Geometry check sheet. Reference: drawing and pictorial views, mm from the part's lowest x, y, z. Coordinates: 2 decimals unless noted, no trailing zeros. Loops run counter-clockwise (first coordinate to the right, second up) from the corner with the lowest first, then second, coordinate; pieces in that order, holes last. Notation, with made-up numbers: (76.25, -1.75) -> (123.25, -1.75) arc R15 ccw to (123.25, 9.25) -> close; hole circle Ø5 at (88, -30). An arc over 180 degrees is marked (long way). Use one line per item in the form item = value.
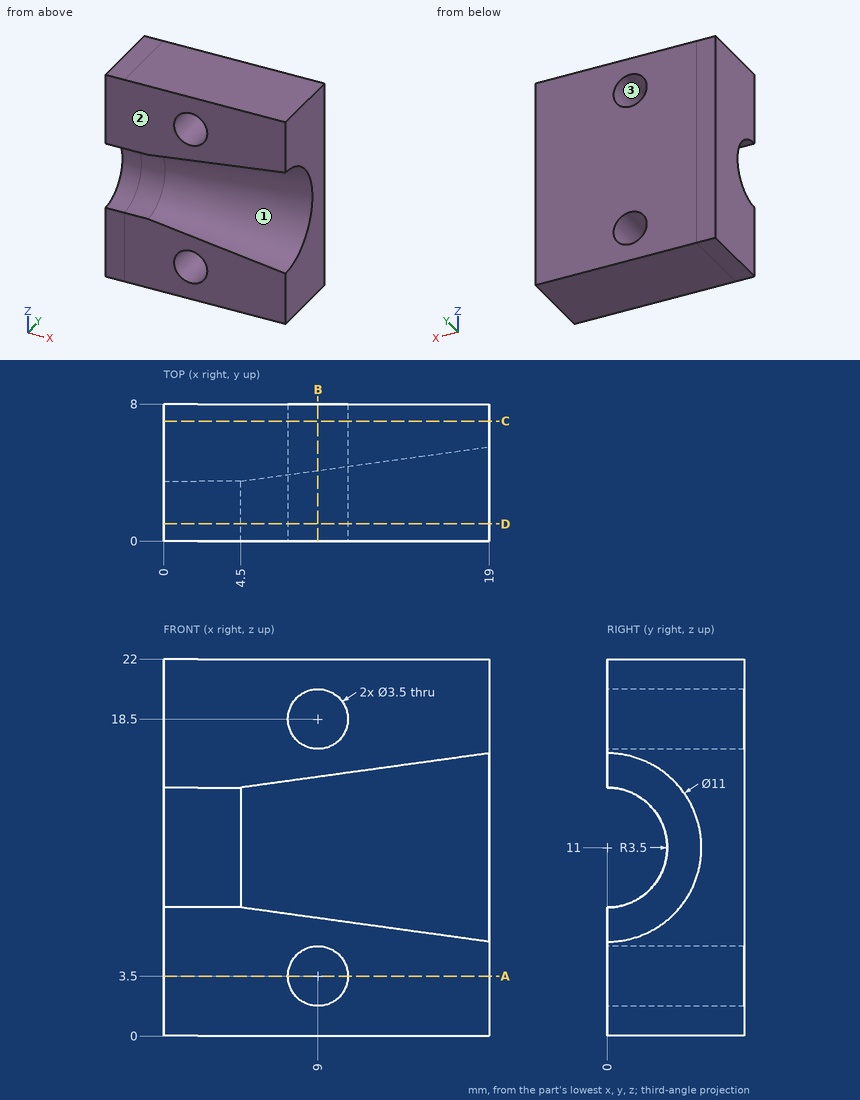
(1) Scan lines: line 1 along Z through (x, y) = (9, 5.75); line 2 along Z through (x, y) = (9.5, 2.5); line 3 along Z through (x, y) = (9, 3). Record each from-to range of solid material in increasing order.
Established:
line_1 = 0 to 1.75, 5.25 to 16.75, 20.25 to 22
line_2 = 0 to 1.82, 5.18 to 7.64, 14.36 to 16.82, 20.18 to 22
line_3 = 0 to 1.75, 5.25 to 8.18, 13.82 to 16.75, 20.25 to 22
(2) Section check D-D, the plane y = 1. Give the number of separate pieces and of enclosed holes in the cut face, plus the area to 3 significant figures.
Established:
separate_pieces = 2
enclosed_holes = 2
area = 241 mm²
(3) Mould release check, pull along X, two halves, no side actions. Record for the marked faces 1, 2 and 3: +X half, -X half, draft (parallel to the pull), parting line (faces both ways), or undercut.
Established:
face_1 = +X half
face_2 = draft
face_3 = undercut
(4) Section check A-A, the plane z = 3.5. Record the boundary of the cut face in (x, y).
Established:
outline = (0, 0) -> (7.25, 0) -> (7.25, 8) -> (0, 8) -> close; (10.75, 0) -> (19, 0) -> (19, 8) -> (10.75, 8) -> close
(5) Go/stop test with flat-tipped pins: P1, Ø4, axis at x = 2.5, z = 10.5, coming from the -Y side; P2, Ø3, axis at x = 9, z = 18.5, coming from the -Y side. Record where each tip stops, or that it passes through.
Established:
P1 = 2.45
P2 = through
(6) Section check C-C, the plane y = 7. Record the boundary of the cut face in (x, z), plus the area to 3 significant figures.
Established:
outline = (0, 0) -> (19, 0) -> (19, 22) -> (0, 22) -> close; hole circle Ø3.5 at (9, 3.5); hole circle Ø3.5 at (9, 18.5)
area = 399 mm²
(7) Section check B-B, the plane x = 9. Record the boundary of the cut face in (y, z), plus the area to 3 significant figures.
Established:
outline = (0, 0) -> (8, 0) -> (8, 1.75) -> (0, 1.75) -> close; (0, 5.25) -> (8, 5.25) -> (8, 16.75) -> (0, 16.75) -> (0, 15.12) arc R4.12 cw to (0, 6.88) -> close; (0, 20.25) -> (8, 20.25) -> (8, 22) -> (0, 22) -> close
area = 93.3 mm²
